Autodesk Inventor part; units mm, degrees
ref_plane "YZ Plane" through (0, 0, 0) normal (1, 0, 0) x (0, 1, 0)
ref_plane "XZ Plane" through (0, 0, 0) normal (0, 1, 0) x (-1, 0, 0)
ref_plane "XY Plane" through (0, 0, 0) normal (0, 0, 1) x (1, 0, 0)
sketch "Esquisse1" plane through (0, 0, 0) normal (0, 0, 1) x (1, 0, 0)
  line L0 (0, 0) -> (-50, 0)
  line L1 (-50, 0) -> (-50, -20)
  line L2 (-50, -20) -> (-79, -20)
  line L3 (-79, -20) -> (-79, 110)
  line L4 (-79, 110) -> (79, 110)
  line L5 (79, 110) -> (79, -20)
  line L6 (79, -20) -> (50, -20)
  line L7 (50, -20) -> (50, 0)
  line L8 (50, 0) -> (0, 0)
  line L9 (-69, 110) -> (-69, 100)
  line L10 (-69, 100) -> (-69, 45) construction
  line L11 (-69, 45) -> (-69, -10) construction
  line L12 (-69, -10) -> (-69, -20)
  line L13 (69, -20) -> (69, -10)
  line L14 (69, -10) -> (69, 45) construction
  line L15 (69, 45) -> (69, 100) construction
  line L16 (69, 100) -> (69, 110)
  circle A0 centre (-69, 100) radius 2
  circle A1 centre (69, 100) radius 2
  circle A2 centre (69, 45) radius 2
  circle A3 centre (-69, 45) radius 2
  circle A4 centre (-69, -10) radius 2
  circle A5 centre (69, -10) radius 2
  line L17 (-69, -10) -> (-79, -10)
  line L18 (69, -10) -> (79, -10)
  line L19 (25, 70) -> (-25, 70) construction
  line L20 (-25, 70) -> (-25, 20) construction
  line L21 (-25, 20) -> (25, 20) construction
  line L22 (25, 20) -> (25, 70) construction
  line L23 (25, 70) -> (-25, 20) construction
  line L24 (-25, 70) -> (25, 20) construction
  line L25 (-69, 45) -> (69, 45) construction
  circle A6 centre (-25, 70) radius 2
  circle A7 centre (25, 70) radius 2
  circle A8 centre (25, 20) radius 2
  circle A9 centre (-25, 20) radius 2
  point P0 (0, 45)
  dimension "d0" = 130
  dimension "d1" = 110
  dimension "d2" = 100
  dimension "d3" = 158
  dimension "d4" = 10
  dimension "d5" = 4
  dimension "d8" = 4
  dimension "d9" = 50
  dimension "d10" = 50
extrude "Extrusion1" add sketch "Esquisse1" against normal blind 5 contours L0 L1 L2 L12 A4 L17 L3 L4 L5 L18 A5 L13 L6 L7 L8 | L2 L3 L17 A4 L12 | L13 A5 L18 L5 L6
properties part number "Plaque avant"
Could you check a few things on this model? Use its own coordinates, in mm. A direction names the side the tool comes from. Give positions to 0.01 mm unless a question says otherwise; leave off trailing zeros. Order: outer loops, then holes, each group sorted by start corner. A loop starts at its lowest first (then second) coordinate and runs counter-clockwise, first axis right, second up.
Item 1: If we section it at B-B, the plane x = -69: Write out the boundary of the cut face in (y, z).
Item 2: I'm going to push a flat-ended pin straight in: pin 1 (6.5 mm diameter, centred on x = -25, y = 70, fed in from +Z). Where does the tip first touch, or does it pass through?
Item 3: I need wall thicknesses on line 1 (X direction, y = 100, z = -2.9); line 2 (Y direction, x = 25, z = -3.8); line 3 (Y direction, x = -69, z = -0.95). Which ranges of each line are inside material? Lowest first, please.
Item 4: If we section it at D-D, the plane z = -3.75: Count the separate pieces of the cut face and the enclosed holes in it, plus the area to 3 significant figures.
Item 5: For faces 1 (the face through (-25, 72, -2)), 2 (the face through (50, -10, -2)), which set-ups out of +Z, -Z, +X, -X, +Y, -Y let a thin tool reach every point of the face, with its end or its side?
Item 6: If we section it at C-C, the plane x = 25: Write out the boundary of the cut face in (y, z).
Item 7: If we mould it in two halves opening along Y, with no side actions, what happens to faces 3 (the face through (1, 0, -2)), 4 (the face through (70.075, 101.686, -2.465)), 5 (the face through (-50, -10, -2)), 6 (the face through (-67.092, -9.399, -2.465))? For each: pulls with the +Y half, pulls with the -Y half, needs draft (parallel to the pull), parting line crosses it, or undercut.
Item 8: If we section it at A-A, the plane y = 70: Write out the boundary of the cut face in (x, z), plus the area to 3 significant figures.
Values:
1. outline: (-20, -5) - (-12, -5) - (-12, 0) - (-20, 0) - close; (-8, -5) - (43, -5) - (43, 0) - (-8, 0) - close; (47, -5) - (98, -5) - (98, 0) - (47, 0) - close; (102, -5) - (110, -5) - (110, 0) - (102, 0) - close
2. pin 1: stops at z = 0
3. line 1: x = -79 to -71, -67 to 67, 71 to 79
3. line 2: y = 0 to 18, 22 to 68, 72 to 110
3. line 3: y = -20 to -12, -8 to 43, 47 to 98, 102 to 110
4. separate pieces: 1
4. enclosed holes: 10
4. area: 18,400 mm2
5. face 1: +Z, -Z
5. face 2: +Z, -Z, -Y
6. outline: (0, -5) - (18, -5) - (18, 0) - (0, 0) - close; (22, -5) - (68, -5) - (68, 0) - (22, 0) - close; (72, -5) - (110, -5) - (110, 0) - (72, 0) - close
7. face 3: pulls with the -Y half
7. face 4: undercut
7. face 5: needs draft
7. face 6: undercut
8. outline: (-79, -5) - (-27, -5) - (-27, 0) - (-79, 0) - close; (-23, -5) - (23, -5) - (23, 0) - (-23, 0) - close; (27, -5) - (79, -5) - (79, 0) - (27, 0) - close
8. area: 750 mm2
